Print and shaded views of the part. All mm, measured from the part's lowest x, y and z. A direction names the side the tool comes from. Round coordinates to 2 decimals unless told otherwise and drop trailing zeros. Loops run counter-clockwise (first coordinate to the right, second up) from the corner with the lowest first, then second, coordinate; pieces in that order, holes last. Notation, with made-up numbers: (11.5, 66.25) -> (22.5, 66.25) arc R21 cw to (22.5, 88.25) -> close; hole circle Ø1 at (85, -32.5). An arc over 180 degrees is marked (long way). Answer as CSV lines item,"result".
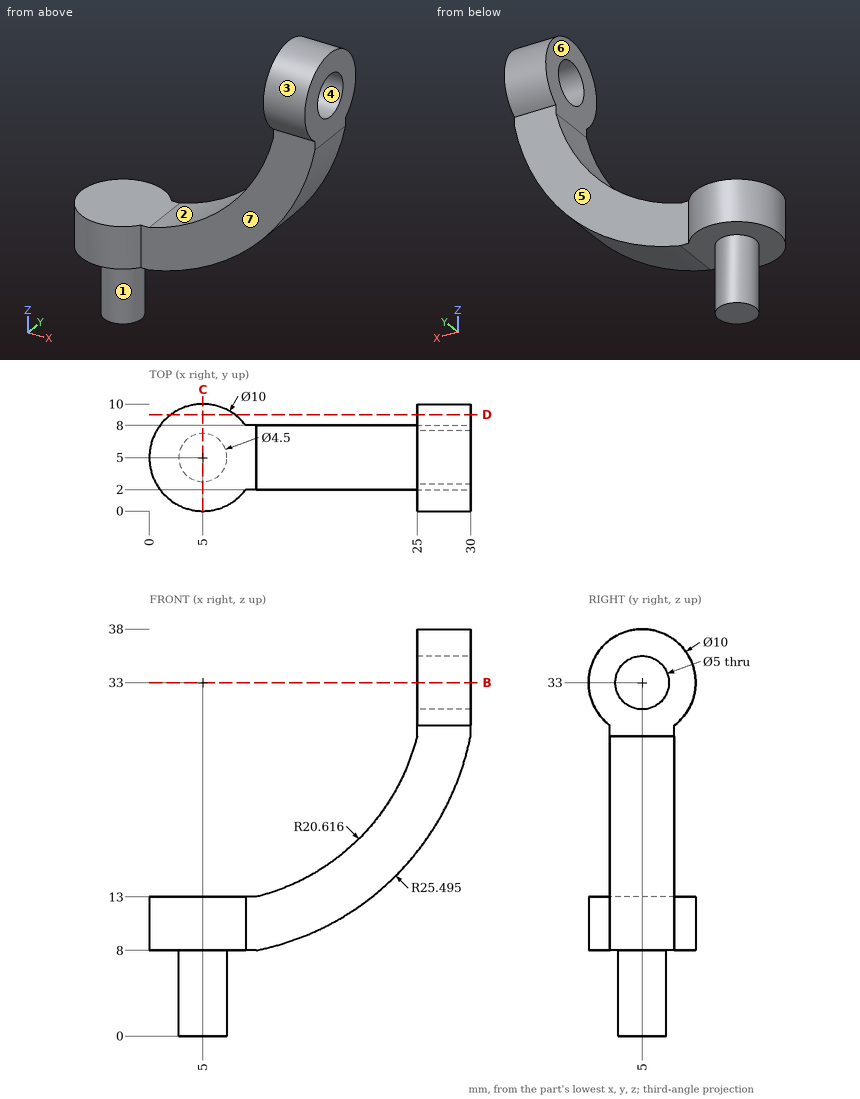
Q1. Saw through at B-B, the plane z = 33. Write the cut outline in (x, y).
Geometry results:
outline,"(25, 0) -> (30, 0) -> (30, 2.5) -> (25, 2.5) -> close; (25, 7.5) -> (30, 7.5) -> (30, 10) -> (25, 10) -> close"
Q2. Saw through at C-C, the plane x = 5. Write the cut outline in (y, z).
Geometry results:
outline,"(0, 8) -> (2.75, 8) -> (2.75, 0) -> (7.25, 0) -> (7.25, 8) -> (10, 8) -> (10, 13) -> (0, 13) -> close"
Q3. Which spindle directions (+Z, -Z, +X, -X, +Y, -Y) get a long thin tool onto all of the face, cutting with end or side? Do the marked faces 5, 6 and 7. Say none if no direction does.
Geometry results:
face 5,"-Z, +X, +Y"
face 6,"+Z, -X, +Y, -Y"
face 7,"-Z, +X, -Y"
Q4. Saw through at D-D, the plane y = 9. Write the cut outline in (x, z), then the cut area to 3 significant figures.
Geometry results:
outline,"(2, 8) -> (8, 8) -> (8, 13) -> (2, 13) -> close; (25, 30) -> (30, 30) -> (30, 36) -> (25, 36) -> close"
area,"60.0 mm2"
Q5. Drill centre lines: line 1 along Y through (x, z) = (26.8, 33); line 2 along Z through (x, y) = (3.25, 9.25); line 3 along X through (y, z) = (4.5, 36.5). Where is each one in solid material? Low to high.
Geometry results:
line 1,"0 to 2.5, 7.5 to 10"
line 2,"8 to 13"
line 3,"25 to 30"
Q6. Two-plate mould, pull along Z, no slides. Class the marked faces 1, 2, 3 and 4: pulls with the +Z half, pulls with the -Z half, needs draft (parallel to the pull), parting line crosses it, or undercut.
Geometry results:
face 1,"needs draft"
face 2,"pulls with the +Z half"
face 3,"parting line crosses it"
face 4,"undercut"
Q7. Drop flat-ended pins along their axis: P1, Ø1, axis at x = 11, z = 9.5, coming from the +Y side; P2, Ø5, axis at x = 4, y = 4, coming from the +Z side; P3, Ø6, axis at y = 6, z = 26.5, coming from the +X side; P4, Ø5, axis at y = 6.5, z = 32, coming from the -X side. Give the stop position or say it passes through.
Geometry results:
P1,"y = 8"
P2,"z = 13"
P3,"x = 30"
P4,"x = 25"
